Can you work these out from the model? Positions are in its coordinate system, mm. Round coordinates to 2 decimals unless told otherwise and drop trailing zeros. Loops run counter-clockwise (first coordinate to the right, second up) from the corner with the lowest first, then second, coordinate; pieces in that order, holes last.
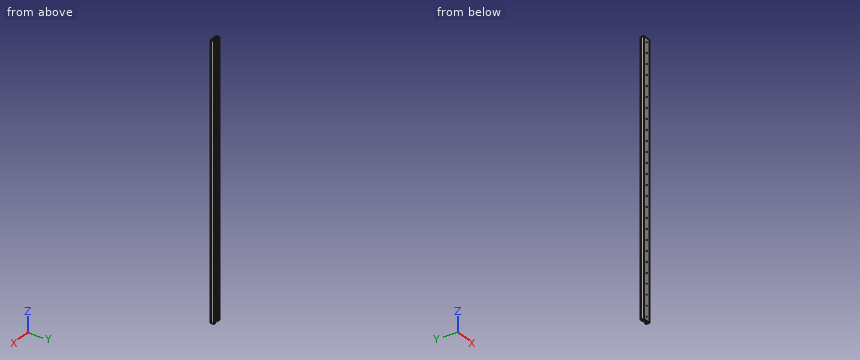
from build123d import *

# Parameters (mm, degrees)
EXTRUDE_1_DEPTH              = 1030
HOLE_WIZARD_M3_1_D           = 3.5
HOLE_WIZARD_M3_1_DEPTH       = 3
HOLE_WIZARD_M3_1_CBORE_D     = 6
HOLE_WIZARD_M3_1_CBORE_DEPTH = 2


with BuildPart() as part:
    # 草图1 → 凸台-拉伸1 (new body)
    with BuildSketch(Plane(origin=(0, 0, -515), x_dir=(-1, 0, 0), z_dir=(0, 0, -1))):
        with BuildLine():
            Line((15, -5.25), (15, 5.25))
            ThreePointArc((15, 5.25), (14.707106781, 5.957106781), (14, 6.25))
            Line((14, 6.25), (6.6, 6.25))
            ThreePointArc((6.6, 6.25), (6.246446609, 6.103553391), (6.1, 5.75))
            Line((6.1, 5.75), (6.1, 3.45))
            ThreePointArc((6.1, 3.45), (6.158578644, 3.308578644), (6.3, 3.25))
            Line((6.3, 3.25), (10, 3.25))
            ThreePointArc((10, 3.25), (10.707106781, 2.957106781), (11, 2.25))
            Line((11, 2.25), (11, -2.25))
            ThreePointArc((11, -2.25), (10.707106781, -2.957106781), (10, -3.25))
            Line((10, -3.25), (-10, -3.25))
            ThreePointArc((-10, -3.25), (-10.707106781, -2.957106781), (-11, -2.25))
            Line((-11, -2.25), (-11, 2.25))
            ThreePointArc((-11, 2.25), (-10.707106781, 2.957106781), (-10, 3.25))
            Line((-10, 3.25), (-6.3, 3.25))
            ThreePointArc((-6.3, 3.25), (-6.158578644, 3.308578644), (-6.1, 3.45))
            Line((-6.1, 3.45), (-6.1, 5.75))
            ThreePointArc((-6.1, 5.75), (-6.246446609, 6.103553391), (-6.6, 6.25))
            Line((-6.6, 6.25), (-14, 6.25))
            ThreePointArc((-14, 6.25), (-14.707106781, 5.957106781), (-15, 5.25))
            Line((-15, 5.25), (-15, -5.25))
            ThreePointArc((-15, -5.25), (-14.707106781, -5.957106781), (-14, -6.25))
            Line((-14, -6.25), (14, -6.25))
            ThreePointArc((14, -6.25), (14.707106781, -5.957106781), (15, -5.25))
        make_face()
    extrude(amount=-EXTRUDE_1_DEPTH)

    # M3 六角头机械螺钉的柱形沉头孔1
    with Locations(Plane(origin=(0, -3.25, 0), x_dir=(1, 0, 0), z_dir=(0, 1, 0))):
        with Locations((0, -500), (0, -460), (0, -420), (0, -380), (0, -340), (0, -300), (0, -260), (0, -220), (0, -180), (0, -140), (0, 20), (0, 60), (0, 100), (0, 140), (0, 180), (0, 220), (0, 260), (0, 300), (0, 340), (0, 380), (0, 420), (0, 460), (0, 500), (0, -100), (0, -60), (0, -20)):
            CounterBoreHole(HOLE_WIZARD_M3_1_D / 2, HOLE_WIZARD_M3_1_CBORE_D / 2, HOLE_WIZARD_M3_1_CBORE_DEPTH, depth=HOLE_WIZARD_M3_1_DEPTH)


solid = part.part
(1) If we section it at A-A, the plane z = -127.5: List the corners of the cut face in (x, y) for me.
Worked answers:
outline: (-15, -5.25) arc R1 ccw to (-14, -6.25) - (14, -6.25) arc R1 ccw to (15, -5.25) - (15, 5.25) arc R1 ccw to (14, 6.25) - (6.6, 6.25) arc R0.5 ccw to (6.1, 5.75) - (6.1, 3.45) arc R0.2 ccw to (6.3, 3.25) - (10, 3.25) arc R1 cw to (11, 2.25) - (11, -2.25) arc R1 cw to (10, -3.25) - (-10, -3.25) arc R1 cw to (-11, -2.25) - (-11, 2.25) arc R1 cw to (-10, 3.25) - (-6.3, 3.25) arc R0.2 ccw to (-6.1, 3.45) - (-6.1, 5.75) arc R0.5 ccw to (-6.6, 6.25) - (-14, 6.25) arc R1 ccw to (-15, 5.25) - close
(2) If I drill on line 1 (X direction, y = 5.5, z = 46.5); line 2 (X direction, y = -4.5, z = -500); line 3 (Y direction, x = -7, z = 245), over which ranges is the centre line in solid material (lowest first)?
Worked answers:
line 1: x = -14.97 to -6.1, 6.1 to 14.97
line 2: x = -15 to -3, 3 to 15
line 3: y = -6.25 to -3.25, 3.25 to 6.25
(3) Will these pins go through, and if not, where does the flat tip stop? P1, Ø8, axis at x = 0, z = -300, coming from the +Y side; P2, Ø4, axis at x = 0, z = 100, coming from the +Y side; P3, Ø1.5, axis at x = 5.5, z = 362, coming from the +Y side.
Worked answers:
P1: stops at y = -3.25
P2: stops at y = -5.25
P3: stops at y = 6.11
